from build123d import *

# Parameters (mm, degrees)
F1_DEPTH = 10
F2_SIZE  = 1.99999
F3_R     = 1.5
F4_DEPTH = 15
F5_R     = 1.5
F6_DEPTH = 15


# Not quite as in the source:
# - a fillet or chamfer is up to 0.001 mm smaller than in the source, because OpenCascade refuses the exact size


with BuildPart() as f1:
    # F0 (on Top) → F1 (new body)
    with BuildSketch(Plane.XY):
        Polygon((-15.3143769915, 8.338528797), (-25.3143769915, 8.338528797), (-25.3143769915, -1.661471203), (-15.3143769915, -1.661471203), (-15.3143769915, 0.338528797), (26.6856230085, 0.338528797), (26.6856230085, -1.661471203), (36.6856230085, -1.661471203), (36.6856230085, 8.338528797), (26.6856230085, 8.338528797), (26.6856230085, 6.338528797), (-15.3143769915, 6.338528797), align=None)
    extrude(amount=F1_DEPTH)

    # F2 (size 2 in the source; OpenCascade refuses exactly that, so slightly less here)
    f2_edges = [f1.edges().sort_by_distance(p)[0] for p in [
        (-15.314377, 8.338529, 5),
        (26.685623, 8.338529, 5),
        (-15.314377, -1.661471, 5),
        (26.685623, -1.661471, 5),
    ]]
    chamfer(f2_edges, length=F2_SIZE)

    # F3 (on face) → F4 (cut)
    with BuildSketch(Plane.YZ.offset(36.6856230085)):
        with Locations((3.338528797, 5)):
            Circle(F3_R)
    extrude(amount=-F4_DEPTH, mode=Mode.SUBTRACT)

    # F5 (on face) → F6 (cut)
    with BuildSketch(Plane(origin=(-25.3143769915, 0, 0), x_dir=(0, -1, 0), z_dir=(-1, 0, 0))):
        with Locations((-3.338528797, 5)):
            Circle(F5_R)
    extrude(amount=-F6_DEPTH, mode=Mode.SUBTRACT)


solid = f1.part
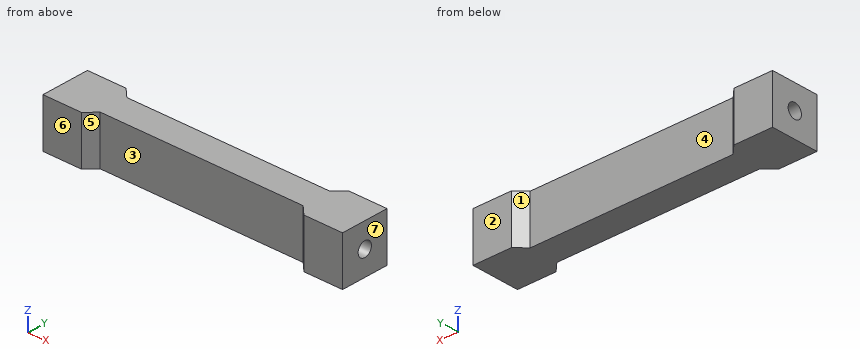
The model under review builds one solid part; all positions refer to its coordinate system, in mm. Face numbers are marked on the shaded views. A direction names the side the tool comes from. Give positions to 0.01 mm unless a question says otherwise; leave off trailing zeros. Order: outer loops, then holes, each group sorted by start corner. A loop starts at its lowest first (then second) coordinate and runs counter-clockwise, first axis right, second up. Notation, with made-up numbers: M 17.5,-0.5 L 41.5,-0.5 A10 cw 41.5,11.5 Z; hole C 37,-21.5 d6. An arc over 180 degrees is marked long. Answer in a Markdown table with one row per item. Add a question column.
1. For pin 1 Ø1.5 at (x, z) = (-3.5, 7) entering from +Y; pin 2 Ø3 at (x, z) = (1.5, 3) entering from -Y; pin 3 Ø0.9 at (y, z) = (4, 4.5) entering from +X, all flat-tipped, find the tip position at first contact; note any pin that passes through.
2. Machinability: for the marked faces 1, 2 and 3, which of the approach directions +Z, -Z, +X, -X, +Y, -Y give a long, thin tool a straight path to every point of the face, cutting with its end or side? Answer none if there is none.
3. Add section B-B on y = -1. State the section outline as (x, z) points.
4. Add section C-C on x = 17. State the section outline as (y, z) points, plus the area to 3 significant figures.
5. To check wall thickness, follow line 1 along X through (y, z) = (-1, 6); line 2 along Y through (x, z) = (16, 5); line 3 along X through (y, z) = (6.5, 6.25). State the ranges of each line that lie inside material, in increasing order.
6. Mouldability with a two-part tool opening along X and no side actions: class the marked faces 4, 5, 6 and 7 as released by +X, released by -X, zero draft, split by the parting line, or undercut.
The answers:
| question | item | result |
|---|---|---|
| 1 | pin 1 | y = 6.34 |
| 1 | pin 2 | y = 0.34 |
| 1 | pin 3 | x = 21.69 |
| 2 | face 1 | +Z, -Z, +Y |
| 2 | face 2 | +Z, -Z, +X, -X, +Y |
| 2 | face 3 | +Z, -Z, -Y |
| 3 | outline | M -25.31,0 L -16.65,0 L -16.65,10 L -25.31,10 Z; M 28.02,0 L 36.69,0 L 36.69,10 L 28.02,10 Z |
| 4 | outline | M 0.34,0 L 6.34,0 L 6.34,10 L 0.34,10 Z |
| 4 | area | 60.0 mm2 |
| 5 | line 1 | -25.31 to -16.65, 28.02 to 36.69 |
| 5 | line 2 | 0.34 to 6.34 |
| 5 | line 3 | -25.31 to -15.48, 26.85 to 36.69 |
| 6 | face 4 | undercut |
| 6 | face 5 | undercut |
| 6 | face 6 | zero draft |
| 6 | face 7 | released by +X |
